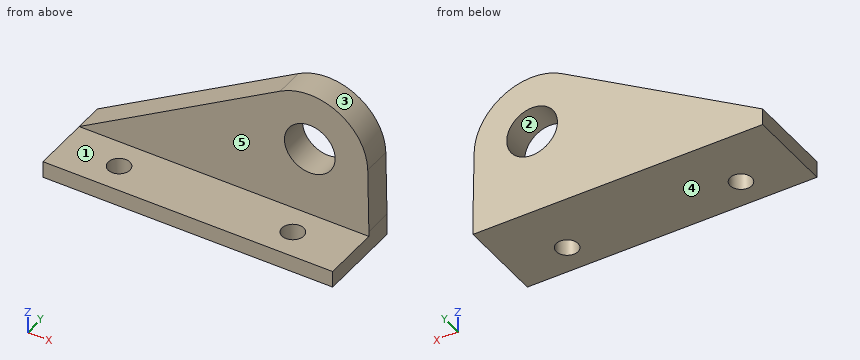
```python
from build123d import *

# Parameters (mm, degrees)
F1_DEPTH = 38.1
F2_DEPTH = 12.7
F3_D     = 22.225
F5_D     = 9.525


with BuildPart() as f1:
    # F0 (on Front) → F1 (new body)
    with BuildSketch(Plane.XZ):
        Polygon((0, 7.2736367583), (0, 0), (127, 0), (127, 7.2736367583), (101.6, 7.2736367583), align=None)
    extrude(amount=F1_DEPTH)

    # F0 (on Front) → F2 (join)
    with BuildSketch(Plane.XZ):
        with BuildLine():
            Line((88.1509339887, 59.4981372414), (0, 7.2736367583))
            Line((0, 7.2736367583), (101.6, 7.2736367583))
            Line((101.6, 7.2736367583), (127, 7.2736367583))
            Line((127, 7.2736367583), (127, 9.525))
            Line((127, 9.525), (126.4935228461, 38.0955111241))
            ThreePointArc((126.4935228461, 38.0955111241), (113.4775446111, 59.8240110713), (88.1509339887, 59.4981372414))
        make_face()
    extrude(amount=F2_DEPTH)

    # F3 (through all)
    with Locations(Plane(origin=(0, 0, 0), x_dir=(1, 0, 0), z_dir=(0, 1, 0))):
        with Locations((101.097512958, -37.6453092096)):
            Hole(F3_D / 2)

    # F5 (through all)
    with Locations(Plane.XY.offset(7.2736367583)):
        with Locations((25.4, -25.4), (101.6, -25.4)):
            Hole(F5_D / 2)


solid = f1.part
```
The model under review builds one solid part; all positions refer to its coordinate system, in mm. Face numbers are marked on the shaded views. A direction names the side the tool comes from. Round coordinates to 2 decimals unless told otherwise and drop trailing zeros. Write each loop counter-clockwise with the first axis right and the second up, starting at its lowest first coordinate (ties: lowest second). Pieces come first, ordered by that corner, then holes. Notation, with made-up numbers: (18.25, -18.5) - (31.25, -18.5) arc R19 ccw to (31.25, -2.5) - close; hole circle Ø7 at (55.25, 86). An arc over 180 degrees is marked (long way). One line per question, with ' | ' between items.
Item 1: The part is to be moulded in two halves that separate along X. For the marked faces 1, 2 and 3, say which applies: pulls with the +X half, pulls with the -X half, needs draft (parallel to the pull), parting line crosses it, or undercut.
Resolved:
face 1: needs draft | face 2: undercut | face 3: parting line crosses it
Item 2: Add section A-A, the plane y = -25.4. Give the boundary of the cut face in (x, z).
Resolved:
outline: (0, 0) - (20.64, 0) - (20.64, 7.27) - (0, 7.27) - close; (30.16, 0) - (96.84, 0) - (96.84, 7.27) - (30.16, 7.27) - close; (106.36, 0) - (127, 0) - (127, 7.27) - (106.36, 7.27) - close
Item 3: Add section C-C, the plane z = 46. Give the boundary of the cut face in (x, y), then the cut area to 3 significant figures.
Resolved:
outline: (65.37, -12.7) - (93.77, -12.7) - (93.77, 0) - (65.37, 0) - close; (108.42, -12.7) - (125.08, -12.7) - (125.08, 0) - (108.42, 0) - close | area: 572 mm2
Item 4: For P1, Ø6, axis at y = -18, z = 38.5, coming from the -X side; P2, Ø4, axis at x = 93.5, z = 43, coming from the -Y side; P3, Ø12, axis at x = 92.5, y = -19, coming from the +Z side, all flat-tipped, find the tip position at first contact; note any pin that passes through.
Resolved:
P1: passes through | P2: stops at y = -12.7 | P3: stops at z = 7.27
Item 5: Add section B-B, the plane x = 101.6. Give the boundary of the cut face in (y, z), then the cut area to 3 significant figures.
Resolved:
outline: (-38.1, 0) - (-30.16, 0) - (-30.16, 7.27) - (-38.1, 7.27) - close; (-20.64, 0) - (0, 0) - (0, 26.54) - (-12.7, 26.54) - (-12.7, 7.27) - (-20.64, 7.27) - close; (-12.7, 48.75) - (0, 48.75) - (0, 63.04) - (-12.7, 63.04) - close | area: 634 mm2
Item 6: For the marked faces 4 and 5, list the 3-axis set-ups (+Z, -Z, +X, -X, +Y, -Y) from which the entire face can be reached by the end or side of a thin tool; tool diameter is ignored.
Resolved:
face 4: -Z, +X, -X, +Y, -Y | face 5: +Z, +X, -X, -Y
Item 7: To check wall thickness, follow probe 1 along Y at (x, z) = (25.4, 3.25); probe 2 along Z at (x, y) = (49, -20); probe 3 along Y at (x, z) = (65, 37.5). State the ranges of each line that lie inside material, in increasing order.
Resolved:
probe 1: y = -38.1 to -30.16, -20.64 to 0 | probe 2: z = 0 to 7.27 | probe 3: y = -12.7 to 0
Item 8: Add section D-D, the plane x = 25.4. Give the boundary of the cut face in (y, z).
Resolved:
outline: (-38.1, 0) - (-30.16, 0) - (-30.16, 7.27) - (-38.1, 7.27) - close; (-20.64, 0) - (0, 0) - (0, 22.32) - (-12.7, 22.32) - (-12.7, 7.27) - (-20.64, 7.27) - close
